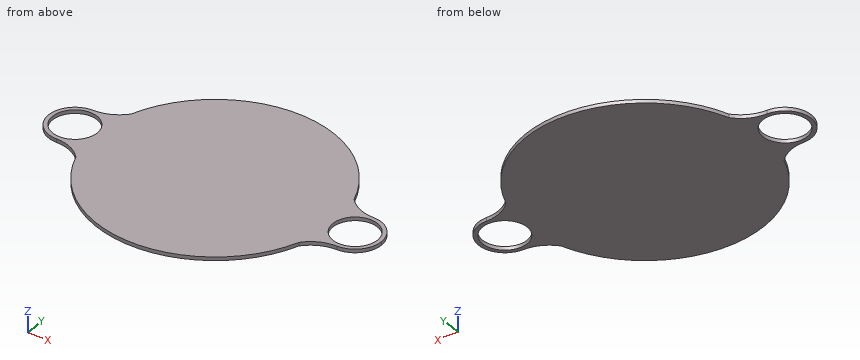
```python
from build123d import *

# Parameters (mm, degrees)
F0_R     = 14.2875
F1_DEPTH = 2.286


with BuildPart() as f1:
    # F0 (on Top) → F1 (new body)
    with BuildSketch(Plane.XY):
        with BuildLine():
            ThreePointArc((-65.750812, -11.062835), (-64.101181, -18.346503), (-61.647349, -25.4))
            ThreePointArc((-61.647349, -25.4), (0, -66.675), (61.647349, -25.4))
            ThreePointArc((61.647349, -25.4), (64.101181, -18.346503), (65.750812, -11.062835))
            ThreePointArc((65.750812, -11.062835), (68.947885, -16.404785), (73.286413, -20.869634))
            ThreePointArc((73.286413, -20.869634), (74.768645, -14.69999), (75.732435, -8.428417))
            ThreePointArc((75.732435, -8.428417), (73.4695, 0), (75.732435, 8.428417))
            ThreePointArc((75.732435, 8.428417), (74.768645, 14.69999), (73.286413, 20.869634))
            ThreePointArc((73.286413, 20.869634), (68.947885, 16.404785), (65.750812, 11.062835))
            ThreePointArc((65.750812, 11.062835), (64.101181, 18.346503), (61.647349, 25.4))
            ThreePointArc((61.647349, 25.4), (0, 66.675), (-61.647349, 25.4))
            ThreePointArc((-61.647349, 25.4), (-64.101181, 18.346503), (-65.750812, 11.062835))
            ThreePointArc((-65.750812, 11.062835), (-66.675, 0), (-65.750812, -11.062835))
        make_face()
        with BuildLine():
            ThreePointArc((-90.297, -16.8275), (-81.890587, -14.577276), (-75.732435, -8.428417))
            ThreePointArc((-75.732435, -8.428417), (-74.045078, -4.363459), (-73.4695, 0))
            ThreePointArc((-73.4695, 0), (-74.045078, 4.363459), (-75.732435, 8.428417))
            ThreePointArc((-75.732435, 8.428417), (-81.890587, 14.577276), (-90.297, 16.8275))
            ThreePointArc((-90.297, 16.8275), (-107.1245, 0), (-90.297, -16.8275))
        make_face()
        with Locations((-90.297, 0)):
            Circle(F0_R, mode=Mode.SUBTRACT)
        with BuildLine():
            ThreePointArc((-75.732435, 8.428417), (-74.768645, 14.69999), (-73.286413, 20.869634))
            ThreePointArc((-73.286413, 20.869634), (-72.599578, 23.146086), (-71.842049, 25.4))
            ThreePointArc((-71.842049, 25.4), (-80.137688, 19.107685), (-90.297, 16.8275))
            ThreePointArc((-90.297, 16.8275), (-81.890587, 14.577276), (-75.732435, 8.428417))
        make_face()
        with BuildLine():
            ThreePointArc((-71.842049, -25.4), (-72.599578, -23.146086), (-73.286413, -20.869634))
            ThreePointArc((-73.286413, -20.869634), (-74.768645, -14.69999), (-75.732435, -8.428417))
            ThreePointArc((-75.732435, -8.428417), (-81.890587, -14.577276), (-90.297, -16.8275))
            ThreePointArc((-90.297, -16.8275), (-80.137688, -19.107685), (-71.842049, -25.4))
        make_face()
        with BuildLine():
            ThreePointArc((-73.286413, -20.869634), (-68.947885, -16.404785), (-65.750812, -11.062835))
            ThreePointArc((-65.750812, -11.062835), (-66.675, 0), (-65.750812, 11.062835))
            ThreePointArc((-65.750812, 11.062835), (-68.947885, 16.404785), (-73.286413, 20.869634))
            ThreePointArc((-73.286413, 20.869634), (-74.768645, 14.69999), (-75.732435, 8.428417))
            ThreePointArc((-75.732435, 8.428417), (-74.045078, 4.363459), (-73.4695, 0))
            ThreePointArc((-73.4695, 0), (-74.045078, -4.363459), (-75.732435, -8.428417))
            ThreePointArc((-75.732435, -8.428417), (-74.768645, -14.69999), (-73.286413, -20.869634))
        make_face()
        with BuildLine():
            ThreePointArc((-73.286413, 20.869634), (-68.947885, 16.404785), (-65.750812, 11.062835))
            ThreePointArc((-65.750812, 11.062835), (-64.101181, 18.346503), (-61.647349, 25.4))
            ThreePointArc((-61.647349, 25.4), (0, 66.675), (61.647349, 25.4))
            ThreePointArc((61.647349, 25.4), (64.101181, 18.346503), (65.750812, 11.062835))
            ThreePointArc((65.750812, 11.062835), (68.947885, 16.404785), (73.286413, 20.869634))
            ThreePointArc((73.286413, 20.869634), (72.599578, 23.146086), (71.842049, 25.4))
            ThreePointArc((71.842049, 25.4), (0, 76.2), (-71.842049, 25.4))
            ThreePointArc((-71.842049, 25.4), (-72.599578, 23.146086), (-73.286413, 20.869634))
        make_face()
        with BuildLine():
            ThreePointArc((61.647349, -25.4), (0, -66.675), (-61.647349, -25.4))
            ThreePointArc((-61.647349, -25.4), (-64.101181, -18.346503), (-65.750812, -11.062835))
            ThreePointArc((-65.750812, -11.062835), (-68.947885, -16.404785), (-73.286413, -20.869634))
            ThreePointArc((-73.286413, -20.869634), (-72.599578, -23.146086), (-71.842049, -25.4))
            ThreePointArc((-71.842049, -25.4), (0, -76.2), (71.842049, -25.4))
            ThreePointArc((71.842049, -25.4), (72.599578, -23.146086), (73.286413, -20.869634))
            ThreePointArc((73.286413, -20.869634), (68.947885, -16.404785), (65.750812, -11.062835))
            ThreePointArc((65.750812, -11.062835), (64.101181, -18.346503), (61.647349, -25.4))
        make_face()
        with BuildLine():
            ThreePointArc((73.286413, 20.869634), (74.768645, 14.69999), (75.732435, 8.428417))
            ThreePointArc((75.732435, 8.428417), (81.890587, 14.577276), (90.297, 16.8275))
            ThreePointArc((90.297, 16.8275), (80.137688, 19.107685), (71.842049, 25.4))
            ThreePointArc((71.842049, 25.4), (72.599578, 23.146086), (73.286413, 20.869634))
        make_face()
        with BuildLine():
            ThreePointArc((75.732435, -8.428417), (74.768645, -14.69999), (73.286413, -20.869634))
            ThreePointArc((73.286413, -20.869634), (72.599578, -23.146086), (71.842049, -25.4))
            ThreePointArc((71.842049, -25.4), (80.137688, -19.107685), (90.297, -16.8275))
            ThreePointArc((90.297, -16.8275), (81.890587, -14.577276), (75.732435, -8.428417))
        make_face()
        with BuildLine():
            ThreePointArc((75.732435, 8.428417), (73.4695, 0), (75.732435, -8.428417))
            ThreePointArc((75.732435, -8.428417), (81.890587, -14.577276), (90.297, -16.8275))
            ThreePointArc((90.297, -16.8275), (102.195839, -11.898839), (107.1245, 0))
            ThreePointArc((107.1245, 0), (102.195839, 11.898839), (90.297, 16.8275))
            ThreePointArc((90.297, 16.8275), (81.890587, 14.577276), (75.732435, 8.428417))
        make_face()
        with Locations((90.297, 0)):
            Circle(F0_R, mode=Mode.SUBTRACT)
    extrude(amount=F1_DEPTH)


solid = f1.part
```
CAD build for the part. Positions are in the model's coordinates, mm. Coordinates: 2 decimals unless noted, no trailing zeros. Write each loop counter-clockwise with the first axis right and the second up, starting at its lowest first coordinate (ties: lowest second). Pieces come first, ordered by that corner, then holes. Notation, with made-up numbers: (43.25, 60.5) -> (90.25, 60.5) arc R19 ccw to (90.25, 75.5) -> close; hole circle Ø4 at (10.5, 21.5). An arc over 180 degrees is marked (long way). Return JSON: item names as keys, results as strings. Group by question number.
Q1. Cut at D-D, the plane y = -44. Give the cut face in (x, z).
Q2. Cut at C-C, the plane x = -15. Give the cut face in (y, z).
Q3. Cut at A-A, the plane z = 1. Give the cut face in (x, y) (1 decimal).
Q4. Flat gauge pin, fed straight in: pin 1 (1 mm diameter, centred on x = -64.5, z = 1.5, fed in from +Y). Where does the tip first touch, or does it go through?
Q5. Cut at B-B, the plane y = 4. Give the cut face in (x, z), then the cut area to 3 significant figures.
Q6. Drill centre lines: line 1 (X direction, y = 1, z = 0.25); line 2 (X direction, y = -1.5, z = 0.45); line 3 (Y direction, x = 86.5, z = 0.9). Where is each one in solid material? Low to high.
Returned:
{
 "1": {"outline": "(-62.21, 0) -> (62.21, 0) -> (62.21, 2.29) -> (-62.21, 2.29) -> close"},
 "2": {"outline": "(-74.71, 0) -> (74.71, 0) -> (74.71, 2.29) -> (-74.71, 2.29) -> close"},
 "3": {"outline": "(-90.3, -16.8) arc R24.5 cw to (-71.8, -25.4) arc R76.2 ccw to (71.8, -25.4) arc R24.5 cw to (90.3, -16.8) arc R16.8 ccw to (107.1, 0) arc R16.8 ccw to (90.3, 16.8) arc R24.5 cw to (71.8, 25.4) arc R76.2 ccw to (-71.8, 25.4) arc R24.5 cw to (-90.3, 16.8) arc R16.8 ccw to start; hole circle Ø28.6 at (-90.3, 0); hole circle Ø28.6 at (90.3, 0)"},
 "4": {"pin 1": "stops at y = 41.36"},
 "5": {"outline": "(-106.64, 0) -> (-104.01, 0) -> (-104.01, 2.29) -> (-106.64, 2.29) -> close; (-76.58, 0) -> (76.58, 0) -> (76.58, 2.29) -> (-76.58, 2.29) -> close; (104.01, 0) -> (106.64, 0) -> (106.64, 2.29) -> (104.01, 2.29) -> close", "area": "362 mm2"},
 "6": {"line 1": "x = -107.09 to -104.55, -76.04 to 76.04, 104.55 to 107.09", "line 2": "x = -107.06 to -104.51, -76.09 to 76.09, 104.51 to 107.06", "line 3": "y = -17.15 to -13.77, 13.77 to 17.15"}
}
